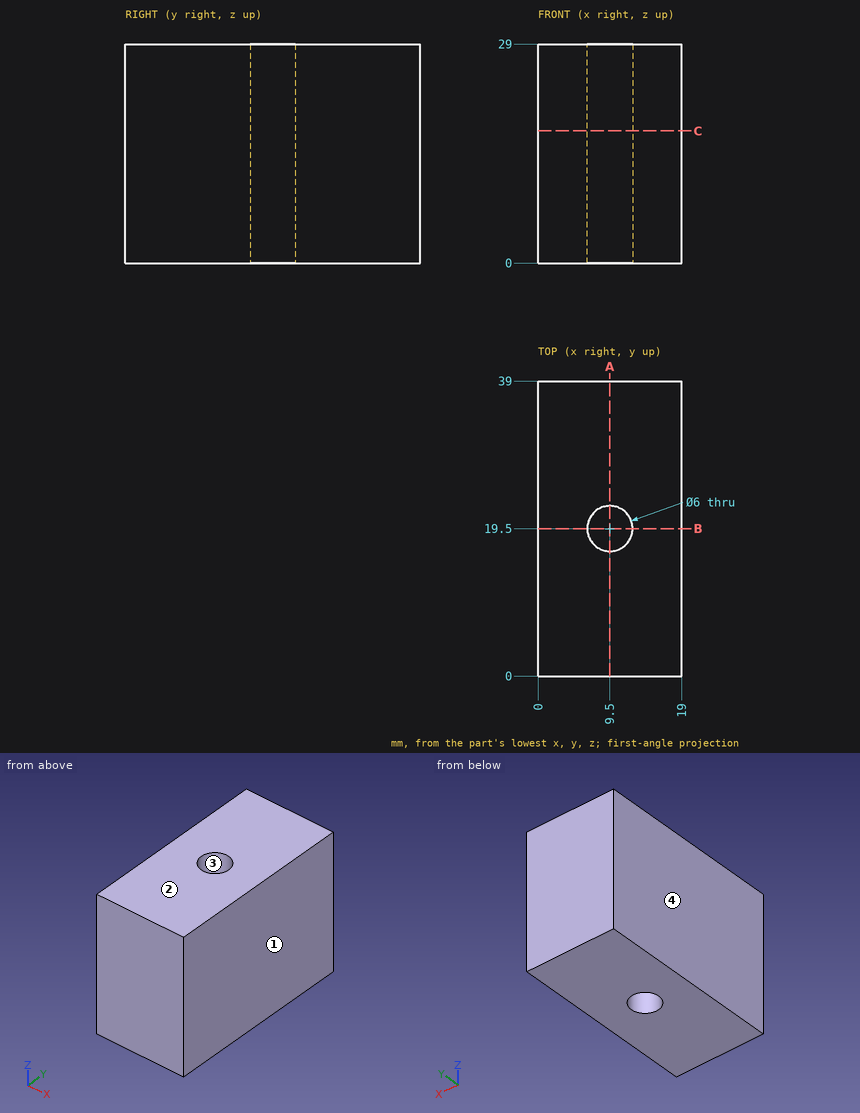
Print and shaded views of the part. All mm, measured from the part's lowest x, y and z. Give positions to 0.01 mm unless a question says otherwise; leave off trailing zeros. Write each loop counter-clockwise with the first axis right and the second up, starting at its lowest first coordinate (ties: lowest second). Pieces come first, ordered by that corner, then holes. Notation, with made-up numbers: (-20.75, -22) - (20.25, -22) arc R26 cw to (20.25, 16) - close; hole circle Ø5 at (13.25, 36.5). An arc over 180 degrees is marked (long way). One line per question, with ' | ' between items. Start each with the question number.
(1) Wall check: line 1 along Y through (x, z) = (9.5, 14.5); line 2 along X through (y, z) = (19.5, 12); line 3 along Y through (x, z) = (10.25, 21). Give the ranges that are in metal, low to high. Write a range as from..to.
(2) Slice it at B-B on y = 19.5. Write the cut outline in (x, z).
(3) Pin check, flat tip, straight feed: P1, Ø2, axis at x = 5.5, y = 31, coming from the -Z side. Stop position of the tip, or through.
(4) Slice it at C-C on z = 17.5. Write the cut outline in (x, y), plus the area to 3 significant figures.
(5) Slice it at A-A on x = 9.5. Write the cut outline in (y, z).
(6) Two-plate mould, pull along X, no slides. Class the marked faces 1, 2, 3 and 4: +X half, -X half, draft (parallel to the pull), parting line (faces both ways), or undercut.
Results below:
1) line 1: 0..16.5, 22.5..39 | line 2: 0..6.5, 12.5..19 | line 3: 0..16.6, 22.4..39
2) outline: (0, 0) - (6.5, 0) - (6.5, 29) - (0, 29) - close; (12.5, 0) - (19, 0) - (19, 29) - (12.5, 29) - close
3) P1: z = 0
4) outline: (0, 0) - (19, 0) - (19, 39) - (0, 39) - close; hole circle Ø6 at (9.5, 19.5) | area: 713 mm^2
5) outline: (0, 0) - (16.5, 0) - (16.5, 29) - (0, 29) - close; (22.5, 0) - (39, 0) - (39, 29) - (22.5, 29) - close
6) face 1: +X half | face 2: draft | face 3: undercut | face 4: -X half
